Part model, mm, in its own coordinate system. Round coordinates to 2 decimals unless told otherwise and drop trailing zeros. Order: outer loops, then holes, each group sorted by start corner. A loop starts at its lowest first (then second) coordinate and runs counter-clockwise, first axis right, second up. Notation, with made-up numbers: (-24.75, -24) -> (-20.75, -24) arc R31 ccw to (-20.75, 11) -> close; hole circle Ø10 at (-12.5, 85.25). An arc over 180 degrees is marked (long way). Use CSV: the item, a comma, the result in double quotes.
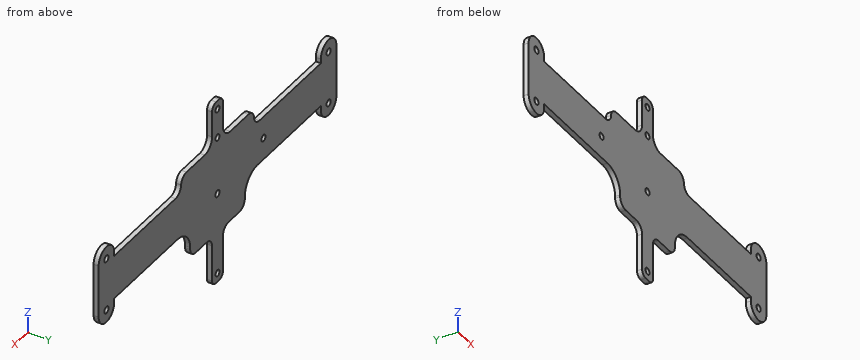
```python
from build123d import *

# Parameters (mm, degrees)
SZKIC1_R                    = 1.15
SZKIC1_R_2                  = 1.150012437
SZKIC1_R_3                  = 1.1
DODANIE_WYCI_GNI_CIE1_DEPTH = 1.7


with BuildPart() as part:
    # Szkic1 → Dodanie-wyciągnięcie1 (new body)
    with BuildSketch(Plane.XZ.offset(-7.087491716)):
        with BuildLine():
            Line((-166.869010382, 45.27), (-166.869010382, 48.27))
            ThreePointArc((-166.869010382, 48.27), (-162.619010382, 52.52), (-158.369010382, 48.27))
            Line((-158.369010382, 48.27), (-158.369010382, 46.77))
            Line((-158.369010382, 46.77), (-124.668997945, 46.77))
            ThreePointArc((-124.668997945, 46.77), (-122.547677602, 47.648679656), (-121.668997945, 49.77))
            Line((-121.668997945, 49.77), (-121.668997945, 49.52))
            ThreePointArc((-121.668997945, 49.52), (-120.790318289, 51.641320344), (-118.668997945, 52.52))
            Line((-118.668997945, 52.52), (-108.668997945, 52.52))
            ThreePointArc((-108.668997945, 52.52), (-105.840570821, 53.691572875), (-104.668997945, 56.52))
            Line((-104.668997945, 56.52), (-104.668997945, 65.32))
            ThreePointArc((-104.668997945, 65.32), (-104.024632864, 66.875634919), (-102.468997945, 67.52))
            Line((-102.468997945, 67.52), (-100.868997945, 67.52))
            ThreePointArc((-100.868997945, 67.52), (-99.313363027, 66.875634919), (-98.668997945, 65.32))
            Line((-98.668997945, 65.32), (-98.668997945, 56.52))
            ThreePointArc((-98.668997945, 56.52), (-97.49742507, 53.691572875), (-94.668997945, 52.52))
            Line((-94.668997945, 52.52), (-84.668997945, 52.52))
            ThreePointArc((-84.668997945, 52.52), (-82.547677602, 51.641320344), (-81.668997945, 49.52))
            Line((-81.668997945, 49.52), (-81.668997945, 49.77))
            ThreePointArc((-81.668997945, 49.77), (-80.790318289, 47.648679656), (-78.668997945, 46.77))
            Line((-78.668997945, 46.77), (-44.968985509, 46.77))
            Line((-44.968985509, 46.77), (-44.968985509, 48.27))
            ThreePointArc((-44.968985509, 48.27), (-40.718985509, 52.52), (-36.468985509, 48.27))
            Line((-36.468985509, 48.27), (-36.468985509, 45.27))
            Line((-36.468985509, 45.27), (-36.468985509, 33.27))
            Line((-36.468985509, 33.27), (-36.468985509, 30.27))
            ThreePointArc((-36.468985509, 30.27), (-40.718985509, 26.02), (-44.968985509, 30.27))
            Line((-44.968985509, 30.27), (-44.968985509, 31.77))
            Line((-44.968985509, 31.77), (-79.668997945, 31.77))
            ThreePointArc((-79.668997945, 31.77), (-84.618745414, 29.719747468), (-86.668997945, 24.77))
            Line((-86.668997945, 24.77), (-86.668997945, 24.17))
            ThreePointArc((-86.668997945, 24.17), (-87.547677602, 22.048679656), (-89.668997945, 21.17))
            Line((-89.668997945, 21.17), (-95.668997945, 21.17))
            ThreePointArc((-95.668997945, 21.17), (-97.790318289, 20.291320344), (-98.668997945, 18.17))
            Line((-98.668997945, 18.17), (-98.668997945, 5.82))
            ThreePointArc((-98.668997945, 5.82), (-99.254784383, 4.405786438), (-100.668997945, 3.82))
            Line((-100.668997945, 3.82), (-102.668997945, 3.82))
            ThreePointArc((-102.668997945, 3.82), (-104.083211508, 4.405786438), (-104.668997945, 5.82))
            Line((-104.668997945, 5.82), (-104.668997945, 18.17))
            ThreePointArc((-104.668997945, 18.17), (-105.547677602, 20.291320344), (-107.668997945, 21.17))
            Line((-107.668997945, 21.17), (-113.668997945, 21.17))
            ThreePointArc((-113.668997945, 21.17), (-115.790318289, 22.048679656), (-116.668997945, 24.17))
            Line((-116.668997945, 24.17), (-116.668997945, 24.77))
            ThreePointArc((-116.668997945, 24.77), (-118.719250477, 29.719747468), (-123.668997945, 31.77))
            Line((-123.668997945, 31.77), (-158.369010382, 31.77))
            Line((-158.369010382, 31.77), (-158.369010382, 30.27))
            ThreePointArc((-158.369010382, 30.27), (-162.619010382, 26.02), (-166.869010382, 30.27))
            Line((-166.869010382, 30.27), (-166.869010382, 33.27))
            Line((-166.869010382, 33.27), (-166.869010382, 45.27))
        make_face()
        with Locations((-162.618997945, 30.27)):
            Circle(SZKIC1_R, mode=Mode.SUBTRACT)
        with Locations((-162.618997945, 48.27)):
            Circle(SZKIC1_R, mode=Mode.SUBTRACT)
        with Locations((-40.718985509, 48.27)):
            Circle(SZKIC1_R_2, mode=Mode.SUBTRACT)
        with Locations((-40.718985509, 30.27)):
            Circle(SZKIC1_R_2, mode=Mode.SUBTRACT)
        with Locations((-101.668997945, 6.82)):
            Circle(SZKIC1_R_3, mode=Mode.SUBTRACT)
        with Locations((-126.869010382, 39.27)):
            Circle(SZKIC1_R_3, mode=Mode.SUBTRACT)
        with Locations((-101.668997945, 54.52)):
            Circle(SZKIC1_R_3, mode=Mode.SUBTRACT)
        with Locations((-101.668997945, 64.52)):
            Circle(SZKIC1_R_3, mode=Mode.SUBTRACT)
        with Locations((-101.668997945, 34.82)):
            Circle(SZKIC1_R, mode=Mode.SUBTRACT)
    extrude(amount=DODANIE_WYCI_GNI_CIE1_DEPTH)


solid = part.part
```
(1) Drop flat-ended pins along their axis: P1, Ø0.5, axis at y = 6.5, z = 9.5, coming from the -X side; P2, Ø0.5, axis at x = -147.5, y = 6.5, coming from the +Z side; P3, Ø0.5, axis at x = -93, y = 6, coming from the -Z side. Give the stop position or say it passes through.
Reply:
P1,"x = -104.67"
P2,"z = 46.77"
P3,"z = 21.17"
(2) Cut at B-B, the plane x = -57. Give the cut face in (y, z).
Reply:
outline,"(5.39, 31.77) -> (7.09, 31.77) -> (7.09, 46.77) -> (5.39, 46.77) -> close"
(3) Cut at C-C, the plane z = 17. Give the cut face in (x, y), then the cut area to 3 significant figures.
Reply:
outline,"(-104.67, 5.39) -> (-98.67, 5.39) -> (-98.67, 7.09) -> (-104.67, 7.09) -> close"
area,"10.2 mm2"
(4) Cut at A-A, the plane y = 6.1. State how many separate pieces and enclosed holes the cut face has, then the cut area to 3 significant figures.
Reply:
separate pieces,"1"
enclosed holes,"9"
area,"2,850 mm2"
(5) Probe probe 1 along X at (y, z) = (5.9, 48); probe 2 along Z at (x, y) = (-95, 6.95); probe 3 along X at (y, z) = (6.55, 35). List the from-to ranges inside material, lowest first. Write a range as [from, to].
Reply:
probe 1,"[-166.87, -163.74], [-161.5, -158.37], [-122.25, -81.09], [-44.97, -41.84], [-39.6, -36.47]"
probe 2,"[21.17, 52.53]"
probe 3,"[-166.87, -102.8], [-100.53, -36.47]"
